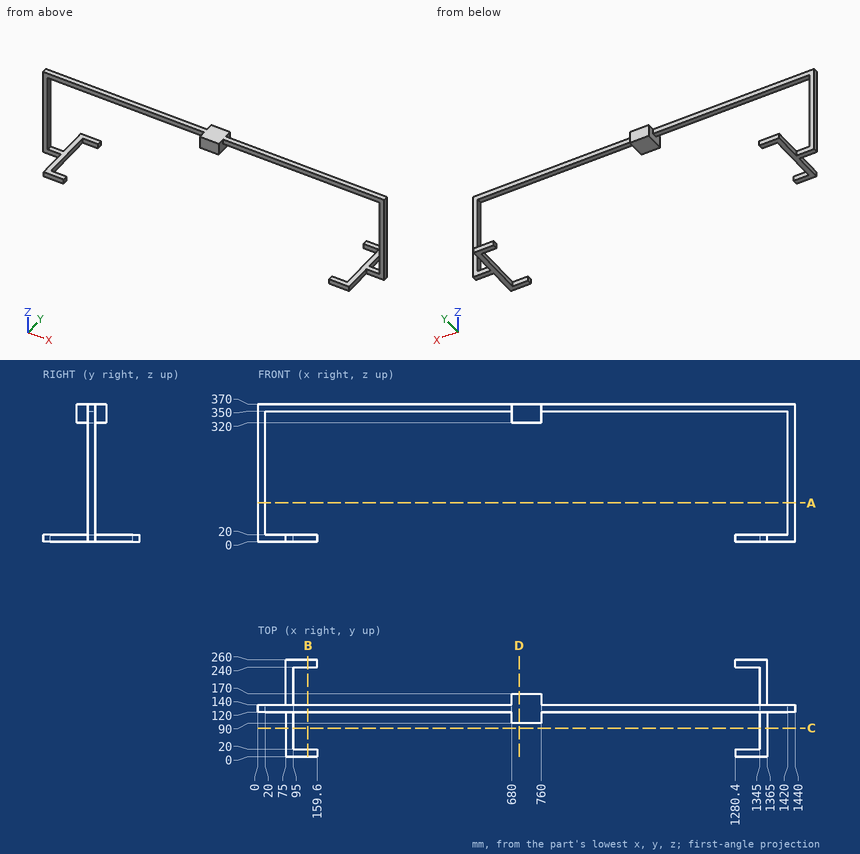
The figure shows three views and two pictorial views of one solid part (mm, origin at its lowest corner). Answer the questions. Coordinates: 2 decimals unless noted, no trailing zeros. Order: outer loops, then holes, each group sorted by start corner. A loop starts at its lowest first (then second) coordinate and runs counter-clockwise, first axis right, second up. Notation, with made-up numbers: M -39.5,26 L -16.5,26 A25 cw -16.5,52 Z; hole C 52.5,66.5 d4. An arc over 180 degrees is marked long. Use CSV: the item, a comma, the result in double quotes.
1) Section B-B on x = 133.5 is taken. Write down the section's boundary in (y, z).
Worked out:
outline,"M 0,0 L 20,0 L 20,20 L 0,20 Z; M 120,350 L 140,350 L 140,370 L 120,370 Z; M 240,0 L 260,0 L 260,20 L 240,20 Z"
2) Flat-ended cylindrical pins translate along their axes: pin 1 Ø22 at (y, z) = (62, 14.5) entering from -X; pin 2 Ø16 at (x, y) = (1220, 129.5) entering from -Z; pin 3 Ø6 at (y, z) = (249.5, 14) entering from +X; pin 4 Ø10 at (x, z) = (1327, 10.5) entering from -Y. Find the tip coordinate at first contact, or state that the pin passes through.
Worked out:
pin 1,"stops at x = 75"
pin 2,"stops at z = 350"
pin 3,"stops at x = 1365"
pin 4,"stops at y = 0"
3) Section A-A on z = 105 is taken. Write down the section's boundary in (x, y), plus the area to 3 significant figures.
Worked out:
outline,"M 0,120 L 20,120 L 20,140 L 0,140 Z; M 1420,120 L 1440,120 L 1440,140 L 1420,140 Z"
area,"800 mm^2"
4) Section C-C on y = 77.5 is taken. Write down the section's boundary in (x, z), plus the area to 3 significant figures.
Worked out:
outline,"M 75,0 L 95,0 L 95,20 L 75,20 Z; M 1345,0 L 1365,0 L 1365,20 L 1345,20 Z"
area,"800 mm^2"
5) Section D-D on x = 700 is taken. Write down the section's boundary in (y, z).
Worked out:
outline,"M 90,320 L 170,320 L 170,370 L 90,370 Z"
6) Consider line 1 (X direction, y = 135.5, z = 252); line 2 (Z direction, x = 896, y = 138); line 3 (Z direction, x = 1352.5, y = 193). Determine where each line is inside the solid, lowest interval first. Write a range as [from, to].
Worked out:
line 1,"x = [0, 20], [1420, 1440]"
line 2,"z = [350, 370]"
line 3,"z = [0, 20]"
